Geometry: see drawing. Coordinates: mm, zero at the bounding-box minimum. A direction names the side the tool comes from. Round coordinates to 2 decimals unless told otherwise and drop trailing zeros. Loops run counter-clockwise (first coordinate to the right, second up) from the corner with the lowest first, then second, coordinate; pieces in that order, holes last. Notation, with made-up numbers: M -3,49 L 40,49 A15 ccw 40,61 Z; hole C 7.5,15 d4. An arc over 180 degrees is marked long. Answer as a JSON object with one key per item and string values.
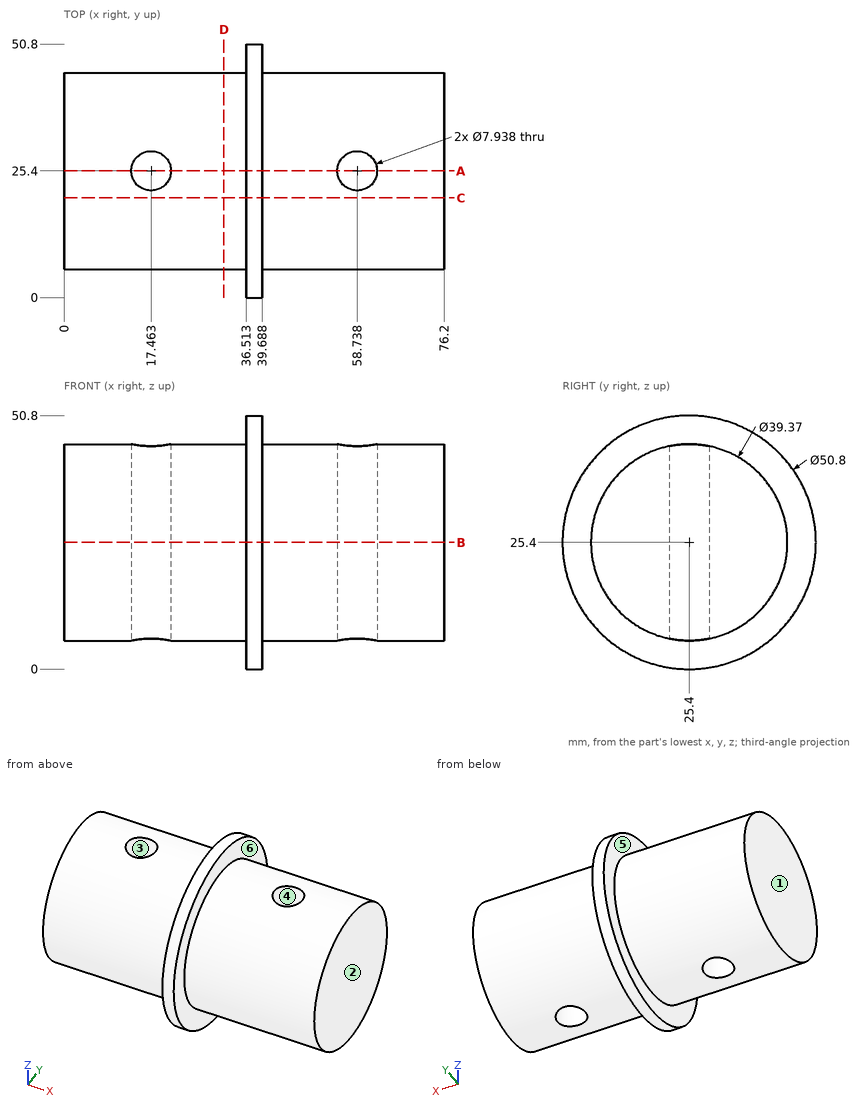
1) Pin query (flat end, axial travel): P1, Ø8, axis at x = 38.5, y = 39.5, coming from the +Z side (1 decimal); P2, Ø9, axis at x = 58.74, y = 25.4, coming from the +Z side (1 decimal); P3, Ø2, axis at x = 58, y = 30.5, coming from the +Z side. Return the tip coordinate at first contact, or that it passes through.
Results:
{"P1": "z = 48.7", "P2": "z = 45.1", "P3": "z = 44.65"}
2) Section query C-C (y = 20). Return the cut outline in (x, z), and give its area (3 significant figures).
Results:
{"outline": "M 0,6.47 L 36.51,6.47 L 36.51,0.58 L 39.69,0.58 L 39.69,6.47 L 76.2,6.47 L 76.2,44.33 L 39.69,44.33 L 39.69,50.22 L 36.51,50.22 L 36.51,44.33 L 0,44.33 Z", "area": "2,920 mm2"}
3) Section query B-B (z = 25.4). Return the cut outline in (x, y) (1 decimal).
Results:
{"outline": "M 0,5.7 L 36.5,5.7 L 36.5,0 L 39.7,0 L 39.7,5.7 L 76.2,5.7 L 76.2,45.1 L 39.7,45.1 L 39.7,50.8 L 36.5,50.8 L 36.5,45.1 L 0,45.1 Z; hole C 17.5,25.4 d7.9; hole C 58.7,25.4 d7.9"}
4) Reachability of the marked faces 4, 5 and 6 from +Z, -Z, +X, -X, +Y, -Y: full face, straight path, thin tool, end or side. Return the list, or none.
Results:
{"face 4": "+Z, -Z", "face 5": "-X", "face 6": "+X"}
5) Pull-direction query (X, two-part tool) for the marked faces 1, 2 and 3; classes: +X half, -X half, draft (parallel to the pull), parting line (faces both ways), or undercut.
Results:
{"face 1": "-X half", "face 2": "+X half", "face 3": "undercut"}
6) Ray query, line 1 (X direction, y = 25.4, z = 35.5); line 2 (X direction, y = 27, z = 23.5) (1 decimal); line 3 (X direction, y = 42, z = 44.5). Return the intervals inside material, ascending.
Results:
{"line 1": "0 to 13.49, 21.43 to 54.77, 62.71 to 76.2", "line 2": "0 to 13.8, 21.1 to 55.1, 62.4 to 76.2", "line 3": "36.51 to 39.69"}
7) Section query A-A (y = 25.4). Return the cut outline in (x, z) (1 decimal).
Results:
{"outline": "M 0,5.7 L 13.5,5.7 L 13.5,45.1 L 0,45.1 Z; M 21.4,5.7 L 36.5,5.7 L 36.5,0 L 39.7,0 L 39.7,5.7 L 54.8,5.7 L 54.8,45.1 L 39.7,45.1 L 39.7,50.8 L 36.5,50.8 L 36.5,45.1 L 21.4,45.1 Z; M 62.7,5.7 L 76.2,5.7 L 76.2,45.1 L 62.7,45.1 Z"}
8) Section query D-D (x = 32). Return the cut outline in (y, z) (1 decimal).
Results:
{"outline": "C 25.4,25.4 d39.4"}
